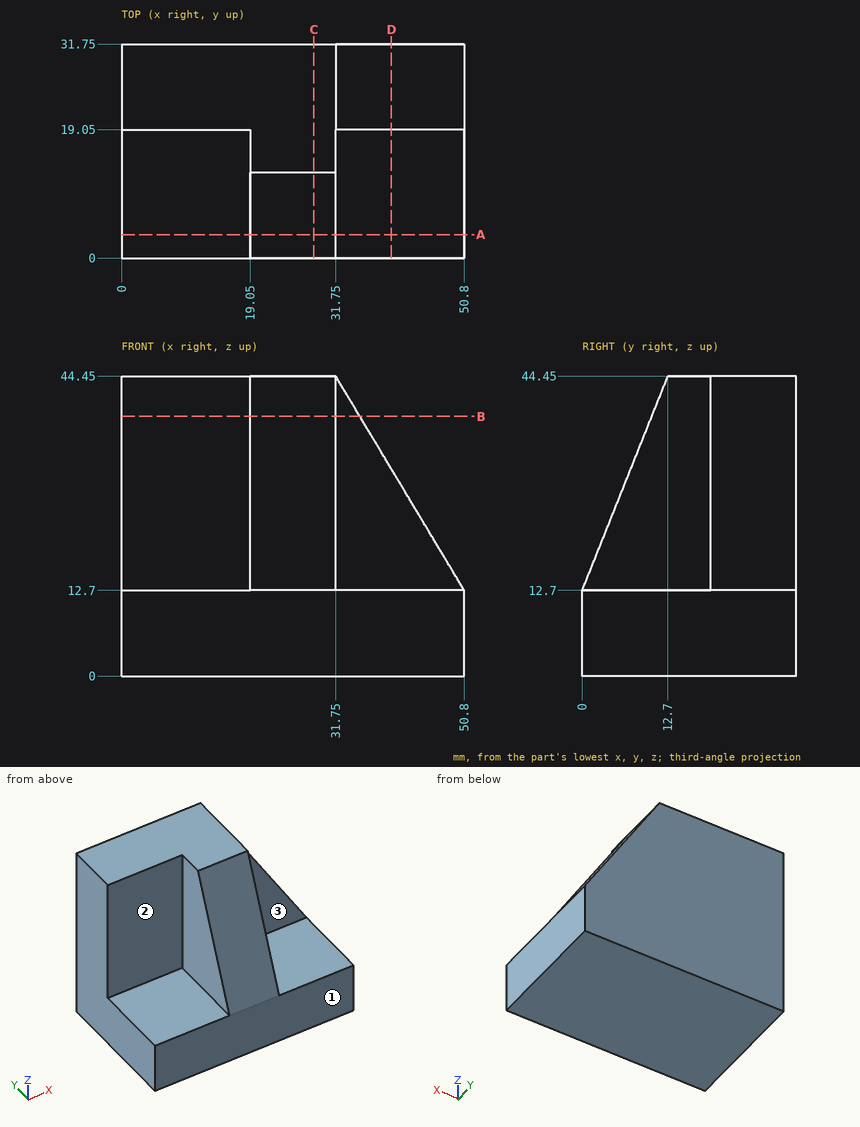
Input: dimensioned drawing with shaded views. Units: mm. Origin: part minimum x, y, z. A direction names the side the tool comes from. Round coordinates to 2 decimals unless told otherwise and drop trailing zeros. Loops run counter-clockwise (first coordinate to the right, second up) from the corner with the lowest first, then second, coordinate; pieces in that order, holes last. Notation, with made-up numbers: (6, -9.5) -> (33, -9.5) arc R31 cw to (33, 14.5) -> close; hole circle Ø7 at (-14.75, 36). An arc over 180 degrees is marked (long way). Answer as a JSON object with one key per item and string values. Group by question number.
1) Ray query, L1, parallel to Y at x = 42.5, z = 14.5; L2, parallel to Z at x = 45, y = 8. Return the intervals inside material, ascending.
2) Section query C-C on x = 28.5. Output: boundary loops of the cut face in (y, z).
3) Pin query (flat end, axial travel): pin 1 (5 mm diameter, centred on y = 6.5, z = 12, fed in from -X); pin 2 (15 mm diameter, centred on x = 11, y = 10.5, fed in from +Z); pin 3 (6 mm diameter, centred on x = 29, z = 37.5, fed in from -Y); pin 4 (6 mm diameter, centred on y = 20.5, z = 19, fed in from +X). Return the tip coordinate at first contact, or that it passes through.
4) Section query A-A on y = 3.5. Output: boundary loops of the cut face in (x, z).
5) Section query B-B on z = 38.5. Output: boundary loops of the cut face in (x, y), plus the area to 3 significant figures.
6) Section query D-D on x = 40. Output: boundary loops of the cut face in (y, z).
7) Reachability of the marked faces 1, 2 and 3 from +Z, -Z, +X, -X, +Y, -Y: full face, straight path, thin tool, end or side. Return the list, or none.
Reply:
{
 "1": {"L1": "y = 19.05 to 31.75", "L2": "z = 0 to 12.7"},
 "2": {"outline": "(0, 0) -> (31.75, 0) -> (31.75, 44.45) -> (12.7, 44.45) -> (0, 12.7) -> close"},
 "3": {"pin 1": "stops at x = 0", "pin 2": "stops at z = 12.7", "pin 3": "stops at y = 8.72", "pin 4": "stops at x = 48.82"},
 "4": {"outline": "(0, 0) -> (50.8, 0) -> (50.8, 12.7) -> (31.75, 12.7) -> (31.75, 21.45) -> (19.05, 21.45) -> (19.05, 12.7) -> (0, 12.7) -> close"},
 "5": {"outline": "(0, 19.05) -> (19.05, 19.05) -> (19.05, 10.32) -> (31.75, 10.32) -> (31.75, 19.05) -> (35.32, 19.05) -> (35.32, 31.75) -> (0, 31.75) -> close", "area": "559 mm2"},
 "6": {"outline": "(0, 0) -> (31.75, 0) -> (31.75, 30.7) -> (19.05, 30.7) -> (19.05, 12.7) -> (0, 12.7) -> close"},
 "7": {"face 1": "+Z, -Z, +X, -X, -Y", "face 2": "+Z, -X, -Y", "face 3": "+Z, +X, -Y"}
}
